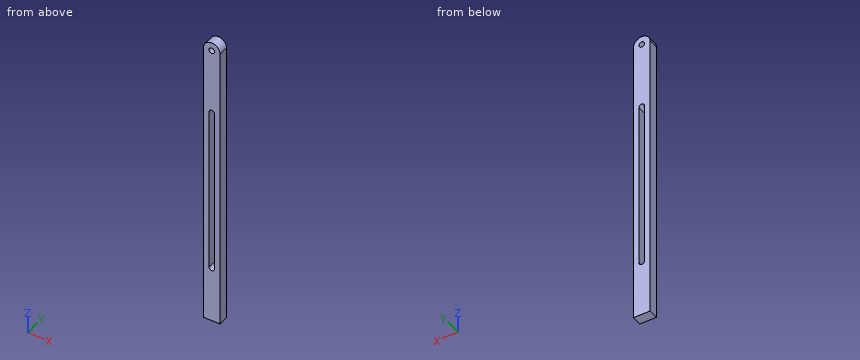
Autodesk Inventor part; units mm, degrees
ref_plane "YZ Plane" through (0, 0, 0) normal (1, 0, 0) x (0, 1, 0)
ref_plane "XZ Plane" through (0, 0, 0) normal (0, 1, 0) x (-1, 0, 0)
ref_plane "XY Plane" through (0, 0, 0) normal (0, 0, 1) x (1, 0, 0)
sketch "Sketch1" plane through (0, 0, 0) normal (0, 1, 0) x (-1, 0, 0)
  line L0 (0, 0) -> (0, -180) construction
  line L1 (5, 0) -> (5, -180)
  line L2 (-5, -180) -> (-5, 0)
  arc A0 (5, 0) -> (-5, 0) centre (0, 0) ccw
  arc A1 (-5, -180) -> (5, -180) centre (0, -180) ccw
  circle A2 centre (0, 0) radius 1.65
  line L3 (0, -40) -> (0, -140) construction
  line L4 (1.65, -40) -> (1.65, -140)
  line L5 (-1.65, -140) -> (-1.65, -40)
  arc A3 (1.65, -40) -> (-1.65, -40) centre (0, -40) ccw
  arc A4 (-1.65, -140) -> (1.65, -140) centre (0, -140) ccw
  point P0 (0, -90)
  point P1 (0, -90)
  dimension "d0" = 180
  dimension "d1" = 10
  dimension "d2" = 3.3
  dimension "d3" = 40
  dimension "d5" = 140
  dimension "d6" = 3.3
extrude "Extrusion1" add sketch "Sketch1" along normal blind 6
sketch "Sketch2" plane through (5, 0, 0) normal (1, 0, 0) x (0, 0, -1)
  line L0 (180, 0) -> (180, 6)
  line L1 (0, 0) -> (180, 0)
  line L2 (180, 0) -> (180, 6)
  line L3 (0, 6) -> (180, 6)
  line L4 (0, 0) -> (0, 6)
  line L5 (180, 0) -> (180, 0)
  line L6 (180, 0) -> (180, 6)
  line L7 (180, 6) -> (180, 6)
  line L8 (180, 0) -> (180, 6)
  line L9 (180, 0) -> (0, 0)
  arc A0 (498.004, -84) -> (180, 0) centre (180, -643.9437) ccw
  line L10 (180, 6) -> (0, 6)
  arc A1 (498.004, -78) -> (180, 6) centre (180, -637.9437) ccw
  line L11 (498.004, -78) -> (498.004, -84)
  line L12 (0, 0) -> (180, 0)
  dimension "d9" = 6
  dimension "d10" = 498.004
  dimension "d11" = 90
extrude "Extrusion2" add sketch "Sketch2" against normal blind 10 contours L0 A1 L11 A0
fillet "Fillet1" radius 2 4 edges at (0, -78, -498.004) (5, -81, -498.004) (-5, -81, -498.004) (0, -84, -498.004)
sketch "Sketch3" plane through (0, 6, 0) normal (0, 1, 0) x (1, 0, 0)
  line L0 (-25.1236, -17.4365) -> (19.1239, -17.4365)
  line L1 (19.1239, -17.4365) -> (19.1239, 173.8027)
  line L2 (19.1239, 173.8027) -> (-25.1236, 173.8027)
  line L3 (-25.1236, 173.8027) -> (-25.1236, -17.4365)
  line L4 (-48.0471, -35.7333) -> (42.457, -35.7333)
  line L5 (42.457, -35.7333) -> (42.457, 337.7497)
  line L6 (42.457, 337.7497) -> (-48.0471, 337.7497)
  line L7 (-48.0471, 337.7497) -> (-48.0471, -35.7333)
  line L8 (-102.0639, -92.3443) -> (98.6132, -92.3443)
  line L9 (98.6132, -92.3443) -> (98.6132, 617.9416)
  line L10 (98.6132, 617.9416) -> (-102.0639, 617.9416)
  line L11 (-102.0639, 617.9416) -> (-102.0639, -92.3443)
  point P0 (0, 0)
extrude "Extrusion3" cut sketch "Sketch3" against normal blind 100 contours L7 L6 L5 L4 | L11 L10 L9 L8
properties part number "Part_8_p3"
Geometry check sheet. Reference: the model listing, model coordinates, mm. Coordinates: 2 decimals unless noted, no trailing zeros. Loops run counter-clockwise (first coordinate to the right, second up) from the corner with the lowest first, then second, coordinate; pieces in that order, holes last. Notation, with made-up numbers: (76.5, -36.5) - (133.5, -36.5) arc R32 cw to (133.5, -6.5) - close; hole circle Ø7 at (10, 29). An arc over 180 degrees is marked (long way). Use one line per item in the form item = value. Start each with the question number.
Item 1: Section check B-B, the plane y = 2.65. Enter the section's corners in (x, z), and give its area (3 significant figures).
Item 2: Thickness scan on probe 1 along Z at (x, y) = (0, 3.65); probe 2 along X at (y, z) = (1.4, -40); probe 3 along Z at (x, y) = (-1.25, 1.85). Record the ranges inside material, lowest first.
Item 3: Section check A-A, the plane x = 0. Enter the section's corners in (y, z), and give its area (3 significant figures).
Item 4: Gauge pin test, flat end, axial feed: pin 1 (2 mm diameter, centred on x = 0, z = 0, fed in from -Y). Record the tip position at first contact, or that the pin passes through.
Item 5: Section check C-C, the plane z = -45. Enter the section's corners in (x, y).
Computed:
q1.outline = (-5, -173.8) - (5, -173.8) - (5, 0) arc R5 ccw to (-5, 0) - close; hole (-1.65, -140) arc R1.65 ccw to (1.65, -140) - (1.65, -40) arc R1.65 ccw to (-1.65, -40) - close; hole circle Ø3.3 at (0, 0)
q1.area = 1,430 mm2
q2.probe_1 = -173.8 to -141.65, -38.35 to -1.65, 1.65 to 5
q2.probe_2 = -5 to -1.65, 1.65 to 5
q2.probe_3 = -173.8 to -141.08, -38.92 to -1.08, 1.08 to 4.84
q3.outline = (0, -173.8) - (6, -173.8) - (6, -141.65) - (0, -141.65) - close; (0, -38.35) - (6, -38.35) - (6, -1.65) - (0, -1.65) - close; (0, 1.65) - (6, 1.65) - (6, 5) - (0, 5) - close
q3.area = 433 mm2
q4.pin_1 = through
q5.outline = (-5, 0) - (-1.65, 0) - (-1.65, 6) - (-5, 6) - close; (1.65, 0) - (5, 0) - (5, 6) - (1.65, 6) - close
